from build123d import *

# Parameters (mm, degrees)
CYLINDER_R        = 8
CYLINDER_DEPTH    = 10
CYLINDER001_R     = 8
CYLINDER001_DEPTH = 10
BOX002_W          = 2
BOX002_H          = 30
BOX002_DEPTH      = 25
FILLET_R          = 10
BOX001_W          = 50
BOX001_H          = 2
BOX001_DEPTH      = 25
FILLET001_R       = 10
BOX_W             = 50
BOX_H             = 30
BOX_DEPTH         = 2


with BuildPart() as cylinder:
    # Cylinder → Cylinder (new body)
    with BuildSketch(Plane(origin=(12.5, 4, 12.5), x_dir=(1, 0, 0), z_dir=(0, -1, 0))):
        Circle(CYLINDER_R)
    extrude(amount=CYLINDER_DEPTH)


with BuildPart() as fusion:
    # Cylinder001 → Cylinder001 (new body)
    with BuildSketch(Plane(origin=(37.5, 4, 12.5), x_dir=(1, 0, 0), z_dir=(0, -1, 0))):
        Circle(CYLINDER001_R)
    extrude(amount=CYLINDER001_DEPTH)

    # Fusion: union Cylinder
    add(cylinder.part)


with BuildPart() as fillet_body:
    # Box002 → Box002 (new body)
    with BuildSketch(Plane(origin=(24, 0, 0), x_dir=(1, 0, 0), z_dir=(0, 0, 1))):
        with Locations((1, 15)):
            Rectangle(BOX002_W, BOX002_H)
    extrude(amount=BOX002_DEPTH)

    # Fillet
    fillet_edges = [fillet_body.edges().sort_by_distance(p)[0] for p in [
        (25, 30, 25),
    ]]
    fillet(fillet_edges, radius=FILLET_R)


with BuildPart() as fillet001:
    # Box001 → Box001 (new body)
    with BuildSketch(Plane.XY):
        with Locations((25, 1)):
            Rectangle(BOX001_W, BOX001_H)
    extrude(amount=BOX001_DEPTH)

    # Fillet001
    fillet001_edges = [fillet001.edges().sort_by_distance(p)[0] for p in [
        (0, 1, 25),
        (50, 1, 25),
    ]]
    fillet(fillet001_edges, radius=FILLET001_R)


with BuildPart() as cut001:
    # Box → Box (new body)
    with BuildSketch(Plane.XY):
        with Locations((25, 15)):
            Rectangle(BOX_W, BOX_H)
    extrude(amount=BOX_DEPTH)

    # Fusion001: union Fillet body, Fillet001
    add(fillet_body.part)
    add(fillet001.part)

    # Cut: cut Fusion
    add(fusion.part, mode=Mode.SUBTRACT)


solid = cut001.part
Build history of the part. All positions in model axes, mm. A direction names the side the tool comes from. Round coordinates to 2 decimals unless told otherwise and drop trailing zeros. Write each loop counter-clockwise with the first axis right and the second up, starting at its lowest first coordinate (ties: lowest second). Pieces come first, ordered by that corner, then holes. Notation, with made-up numbers: (72, 34) - (80, 34) arc R12 cw to (80, 44) - close; hole circle Ø4 at (13.5, 51.5). An arc over 180 degrees is marked (long way). One line per question, with ' | ' between items.
1. Mould opens along Z. For faces 4 (the face through (43.2, 2, 18.5)), 5 (the face through (12, 16, 2)), 6 (the face through (31.151, 1.014, 7.632)) say: released by +Z, released by -Z, zero draft, split by the parting line, or undercut.
Results are:
face 4: zero draft | face 5: released by +Z | face 6: undercut
2. Tool access for faces 1 (the face through (25, 30, 2)), 2 (the face through (26, 16, 13)), 3 (the face through (6, 2, 18)): list every direction of +Z, -Z, +X, -X, +Y, -Y with a clear straight run to the whole face (end or side of a thin tool).
Results are:
face 1: +Z, -Z, +X, -X, +Y | face 2: +Z, +X, +Y | face 3: +Z, -X, +Y
3. Drill centre lines: line 1 along X through (y, z) = (0.7, 12.5); line 2 along Z through (x, y) = (12.5, 0.9); line 3 along Y through (x, z) = (16.5, 23.5). Where is each one in solid material? Low to high. Write a range as from..to.
Results are:
line 1: 0..4.5, 20.5..29.5, 45.5..50 | line 2: 0..4.5, 20.5..25 | line 3: 0..2
4. Drop flat-ended pins along their axis: pin 1 Ø11.5 at (y, z) = (21, 16.5) entering from -X; pin 2 Ø8 at (y, z) = (20, 21.5) entering from +X; pin 3 Ø10 at (x, y) = (40, 15.5) entering from -Z; pin 4 Ø1 at (x, y) = (13, 24) entering from +Z. Give the stop position or say it passes through.
Results are:
pin 1: x = 24 | pin 2: x = 26 | pin 3: z = 0 | pin 4: z = 2
5. Band-saw the part on B-B, the plane z = 12.5. Write the cut outline in (x, y).
Results are:
outline: (0, 0) - (4.5, 0) - (4.5, 2) - (0, 2) - close; (20.5, 0) - (29.5, 0) - (29.5, 2) - (26, 2) - (26, 30) - (24, 30) - (24, 2) - (20.5, 2) - close; (45.5, 0) - (50, 0) - (50, 2) - (45.5, 2) - close
6. Band-saw the part on D-D, the plane y = 7. Write the cut outline in (x, z).
Results are:
outline: (0, 0) - (50, 0) - (50, 2) - (26, 2) - (26, 25) - (24, 25) - (24, 2) - (0, 2) - close
7. Band-saw the part on A-A, the plane x = 12.5. Write the cut outline in (y, z), and give its area (3 significant figures).
Results are:
outline: (0, 0) - (30, 0) - (30, 2) - (2, 2) - (2, 4.5) - (0, 4.5) - close; (0, 20.5) - (2, 20.5) - (2, 25) - (0, 25) - close | area: 74.0 mm^2
8. Band-saw the part on C-C, the plane z = 3. Write the cut outline in (x, y), and give its area (3 significant figures).
Results are:
outline: (0, 0) - (50, 0) - (50, 2) - (26, 2) - (26, 30) - (24, 30) - (24, 2) - (0, 2) - close | area: 156 mm^2
